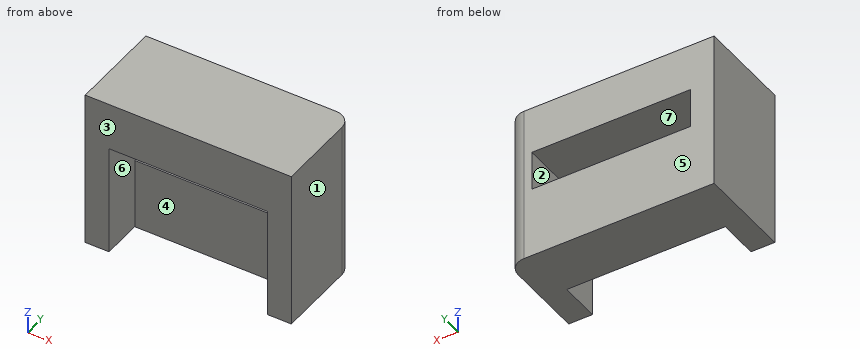
```python
from build123d import *

# Parameters (mm, degrees)
PAD014_DEPTH    = 10
SKETCH_W        = 10
SKETCH_H        = 2.5
POCKET_DEPTH    = 5
SKETCH029_W     = 13
SKETCH029_H     = 3
PAD015_DEPTH    = 3
SKETCH030_W     = 10
SKETCH030_H     = 7
POCKET002_DEPTH = 1


with BuildPart() as obj1:
    # Sketch015 → Pad014 (new body)
    with BuildSketch(Plane.XY):
        with BuildLine():
            Line((10, -9), (10, -15))
            Line((10, -15), (12.625, -15))
            Line((12.625, -15), (12.625, -14.4))
            Line((12.625, -14.4), (11.5, -14.4))
            Line((11.5, -14.4), (11.5, -12.45))
            Line((11.5, -12.45), (21.5, -12.45))
            Line((21.5, -12.45), (21.5, -14.4))
            Line((21.5, -14.4), (20.375, -14.4))
            Line((20.375, -14.4), (20.375, -15))
            Line((20.375, -15), (23, -15))
            Line((23, -15), (23, -10))
            ThreePointArc((23, -10), (22.707107, -9.292893), (22, -9))
            Line((22, -9), (10, -9))
        make_face()
    extrude(amount=PAD014_DEPTH)

    # Sketch (on Face6 of Pad014) → Pocket (cut)
    with BuildSketch(Plane.XZ.offset(12.45)):
        with Locations((16.5, 4.25)):
            Rectangle(SKETCH_W, SKETCH_H)
    extrude(amount=-POCKET_DEPTH, mode=Mode.SUBTRACT)

    # Sketch029 (on Face4 of Pocket) → Pad015 (join)
    with BuildSketch(Plane(origin=(0, 0, 0), x_dir=(1, 0, 0), z_dir=(0, 0, -1))):
        with Locations((16.5, 13.5)):
            Rectangle(SKETCH029_W, SKETCH029_H)
    extrude(amount=-PAD015_DEPTH)

    # Sketch030 (on Face4 of Pad015) → Pocket002 (cut)
    with BuildSketch(Plane.XZ.offset(15)):
        with Locations((16.5, 6.5)):
            Rectangle(SKETCH030_W, SKETCH030_H)
    extrude(amount=-POCKET002_DEPTH, mode=Mode.SUBTRACT)


with BuildPart() as obj2:
    # Part__Mirroring: instance of obj1
    add(obj1.part.mirror(Plane(origin=(0, 0, 72.5), x_dir=(0, 1, 0), z_dir=(0, 0, 1))))


solid = obj2.part
```
Verification items for the finished model (mm, model axes). Face numbers are marked on the shaded views. A direction names the side the tool comes from. Give positions to 0.01 mm unless a question says otherwise; leave off trailing zeros. Loops run counter-clockwise (first coordinate to the right, second up) from the corner with the lowest first, then second, coordinate; pieces in that order, holes last.
1. Go/stop test with a flat-tipped pin: pin 1 Ø5 at (x, z) = (17, 136.5) entering from -Y. Record where the tip stops, or that it passes through.
2. Section check B-B, the plane z = 139.75. Enter the section's corners in (x, y).
3. Set-up check for the marked faces 5, 6 and 7: record each of +Z, -Z, +X, -X, +Y, -Y from which the full face is reachable in a straight line by a thin tool's end or side.
4. Section check A-A, the plane y = -11. Enter the section's corners in (x, z).
5. Section check C-C, the plane x = 13.75. Enter the section's corners in (y, z).
6. Mould release check, pull along X, two halves, no side actions. Record for the marked faces 1, 2, 3 and 4: released by +X, released by -X, zero draft, split by the parting line, or undercut.
7. Section check D-D, the plane y = -13.25. Enter the section's corners in (x, z).
8. Thickness scan on line 1 (Z direction, x = 21, y = -12); line 2 (X direction, y = -13.25, z = 139.5); line 3 (Z direction, x = 15.25, y = -13.5). Record the ranges inside material, lowest first.
Geometry says:
1. pin 1: stops at y = -12.45
2. outline: (10, -15) - (11.5, -15) - (11.5, -9) - (10, -9) - close; (21.5, -15) - (23, -15) - (23, -10) arc R1 ccw to (22, -9) - (21.5, -9) - close
3. face 5: +Z, -Z, +X, -X, +Y
3. face 6: -Y
3. face 7: +Y, -Y
4. outline: (10, 135) - (23, 135) - (23, 145) - (10, 145) - close; hole (11.5, 139.5) - (21.5, 139.5) - (21.5, 142) - (11.5, 142) - close
5. outline: (-15, 142) - (-9, 142) - (-9, 145) - (-15, 145) - close; (-12.45, 135) - (-9, 135) - (-9, 139.5) - (-12.45, 139.5) - close
6. face 1: released by +X
6. face 2: undercut
6. face 3: zero draft
6. face 4: undercut
7. outline: (10, 135) - (11.5, 135) - (11.5, 142) - (21.5, 142) - (21.5, 135) - (23, 135) - (23, 145) - (10, 145) - close
8. line 1: z = 135 to 139.5, 142 to 145
8. line 2: x = 10 to 11.5, 21.5 to 23
8. line 3: z = 142 to 145
